Can you work these out from the drawing? Everything is in mm from the part's minimum corner. A direction names the side the tool comes from. Give positions to 0.01 mm unless a question says otherwise; leave off trailing zeros. Order: outer loops, then holes, each group sorted by start corner. A loop starts at its lowest first (then second) coordinate and runs counter-clockwise, first axis right, second up. Notation, with made-up numbers: (44, -19.75) - (65, -19.75) arc R19 ccw to (65, 8.25) - close; hole circle Ø7 at (-34.5, 48.5). An arc over 180 degrees is marked (long way). Answer as a JSON object with one key per item and string values.
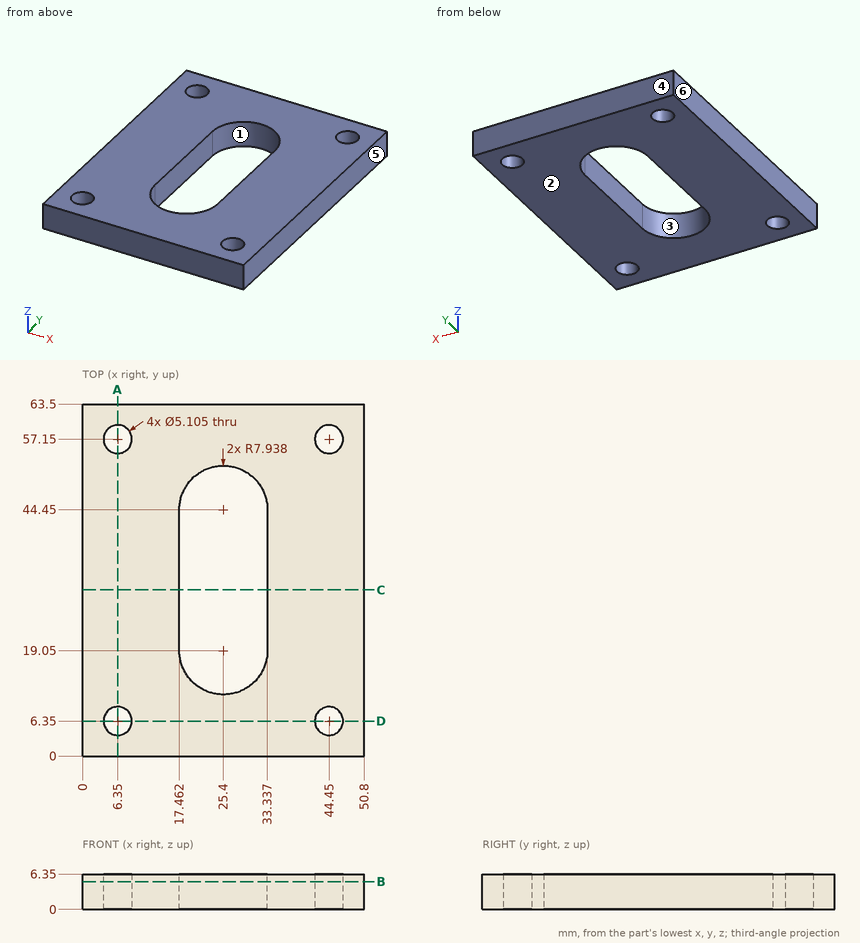
Q1. If we section it at B-B, the plane z = 5: Count the separate pieces of the cut face and the enclosed holes in it, then the cut area to 3 significant figures.
Recorded:
{"separate pieces": "1", "enclosed holes": "5", "area": "2,540 mm^2"}
Q2. I need wall thicknesses on L1, parallel to X at y = 57, z = 2.75; L2, parallel to Y at x = 44.45, z = 3; L3, parallel to X at y = 35, z = 5.75. Which ranges of each line are inside material? Lowest first, please.
Recorded:
{"L1": "x = 0 to 3.8, 8.9 to 41.9, 47 to 50.8", "L2": "y = 0 to 3.8, 8.9 to 54.6, 59.7 to 63.5", "L3": "x = 0 to 17.46, 33.34 to 50.8"}
Q3. If we section it at A-A, the plane x = 6.35: Please give me the cut outline in (y, z).
Recorded:
{"outline": "(0, 0) - (3.8, 0) - (3.8, 6.35) - (0, 6.35) - close; (8.9, 0) - (54.6, 0) - (54.6, 6.35) - (8.9, 6.35) - close; (59.7, 0) - (63.5, 0) - (63.5, 6.35) - (59.7, 6.35) - close"}
Q4. We'd pull the mould along X, two halves only. Please class the marked faces 3, 4, 5 and 6: released by +X, released by -X, zero draft, split by the parting line, or undercut.
Recorded:
{"face 3": "undercut", "face 4": "zero draft", "face 5": "released by +X", "face 6": "released by -X"}
Q5. If we section it at C-C, the plane y = 30: Please give me the cut outline in (x, z).
Recorded:
{"outline": "(0, 0) - (17.46, 0) - (17.46, 6.35) - (0, 6.35) - close; (33.34, 0) - (50.8, 0) - (50.8, 6.35) - (33.34, 6.35) - close"}
Q6. If we section it at D-D, the plane y = 6.35: Please give me the cut outline in (x, z), then the cut area to 3 significant figures.
Recorded:
{"outline": "(0, 0) - (3.8, 0) - (3.8, 6.35) - (0, 6.35) - close; (8.9, 0) - (41.9, 0) - (41.9, 6.35) - (8.9, 6.35) - close; (47, 0) - (50.8, 0) - (50.8, 6.35) - (47, 6.35) - close", "area": "258 mm^2"}
Q7. Which directions (+Z, -Z, +X, -X, +Y, -Y) give clear straight access to the entire face, cutting with the end or side of a thin tool? Please do the marked faces 1 and 2.
Recorded:
{"face 1": "+Z, -Z", "face 2": "-Z, +X, -X, +Y, -Y"}
